from build123d import *

# Parameters (mm, degrees)
F0_W         = 185.6
F0_H         = 105.4
F1_DEPTH     = 6
F2_R         = 22.5
F3_DEPTH     = 25
F4_R         = 2
F5_T1_DEPTH  = 9
F5_S5_W      = 2
F5_S5_H      = 2
F5_T6_DEPTH  = 2
F5_S11_W     = 2
F5_S11_H     = 2
F5_T12_DEPTH = 2
F5_S17_W     = 2
F5_S17_H     = 2
F5_T18_DEPTH = 2
F5_S23_W     = 2
F5_S23_H     = 2
F5_T24_DEPTH = 2


# Not quite as in the source:
# - a fillet or chamfer that OpenCascade refuses, or shapes differently, is made with other operations: its cross-section is extruded or revolved along the edge and cut away or added


with BuildPart() as f1:
    # F0 (on Top) → F1 (new body)
    with BuildSketch(Plane.XY):
        Rectangle(F0_W, F0_H)
    extrude(amount=F1_DEPTH)

    # F2 (on face) → F3 (cut)
    with BuildSketch(Plane.XY.offset(6)):
        with Locations((50.1459216796, 0)):
            Circle(F2_R)
    extrude(amount=-F3_DEPTH, mode=Mode.SUBTRACT)

    # F4
    f4_edges = [f1.edges().sort_by_distance(p)[0] for p in [
        (0, -52.7, 6),
        (92.8, 0, 6),
        (0, 52.7, 6),
        (-92.8, 0, 6),
    ]]
    fillet(f4_edges, radius=F4_R)

    # F5: fillet of radius 2 on 4 edges, made by hand

    # F5_s2 → F5_t1 (cut)
    with BuildSketch(Plane.XY.offset(-5)):
        with BuildLine():
            ThreePointArc((92.8, -50.7), (92.2142135624, -52.1142135624), (90.8, -52.7))
            Line((90.8, -52.7), (92.8, -52.7))
            Line((92.8, -52.7), (92.8, -50.7))
        make_face()
        with BuildLine():
            ThreePointArc((92.8, 50.7), (92.2142135624, 52.1142135624), (90.8, 52.7))
            Line((90.8, 52.7), (92.8, 52.7))
            Line((92.8, 52.7), (92.8, 50.7))
        make_face()
        with BuildLine():
            ThreePointArc((-90.8, 52.7), (-92.2142135624, 52.1142135624), (-92.8, 50.7))
            Line((-92.8, 50.7), (-92.8, 52.7))
            Line((-92.8, 52.7), (-90.8, 52.7))
        make_face()
        with BuildLine():
            ThreePointArc((-90.8, -52.7), (-92.2142135624, -52.1142135624), (-92.8, -50.7))
            Line((-92.8, -50.7), (-92.8, -52.7))
            Line((-92.8, -52.7), (-90.8, -52.7))
        make_face()
    extrude(amount=F5_T1_DEPTH, mode=Mode.SUBTRACT)


with BuildPart() as f5_tool4:
    # F5_s5 → F5_t6 (new body)
    with BuildSketch(Plane.XZ.offset(50.7)):
        with Locations((-91.8, 5)):
            Rectangle(F5_S5_W, F5_S5_H)
    extrude(amount=F5_T6_DEPTH)

    # F5_s7 → F5_t8 (revolve, cut)
    with BuildSketch(Plane(origin=(-90.8, -50.7, 4), x_dir=(0.7071067812, 0, -0.7071067812), z_dir=(-0.7071067812, 0, -0.7071067812))):
        with BuildLine():
            ThreePointArc((0, -2), (2, 0), (0, 2))
            Line((0, 2), (0, -2))
        make_face()
    revolve(axis=Axis((-90.8, -50.7, 4), (0, -1, 0)), mode=Mode.SUBTRACT)


with BuildPart() as f1_1:
    add(f1.part)

    # F5_t3: cut F5_tool4
    add(f5_tool4.part, mode=Mode.SUBTRACT)


with BuildPart() as f5_tool10:
    # F5_s11 → F5_t12 (new body)
    with BuildSketch(Plane.XZ.offset(-50.7)):
        with Locations((-91.8, 5)):
            Rectangle(F5_S11_W, F5_S11_H)
    extrude(amount=-F5_T12_DEPTH)

    # F5_s13 → F5_t14 (revolve, cut)
    with BuildSketch(Plane(origin=(-90.8, 50.7, 4), x_dir=(0.7071067812, 0, -0.7071067812), z_dir=(0.7071067812, 0, 0.7071067812))):
        with BuildLine():
            ThreePointArc((0, -2), (2, 0), (0, 2))
            Line((0, 2), (0, -2))
        make_face()
    revolve(axis=Axis((-90.8, 50.7, 4), (0, 1, 0)), mode=Mode.SUBTRACT)


with BuildPart() as f1_2:
    add(f1_1.part)

    # F5_t9: cut F5_tool10
    add(f5_tool10.part, mode=Mode.SUBTRACT)


with BuildPart() as f5_tool16:
    # F5_s17 → F5_t18 (new body)
    with BuildSketch(Plane.YZ.offset(90.8)):
        with Locations((51.7, 5)):
            Rectangle(F5_S17_W, F5_S17_H)
    extrude(amount=F5_T18_DEPTH)

    # F5_s19 → F5_t20 (revolve, cut)
    with BuildSketch(Plane(origin=(90.8, 50.7, 4), x_dir=(0, -0.7071067812, -0.7071067812), z_dir=(0, -0.7071067812, 0.7071067812))):
        with BuildLine():
            ThreePointArc((0, -2), (2, 0), (0, 2))
            Line((0, 2), (0, -2))
        make_face()
    revolve(axis=Axis((90.8, 50.7, 4), (1, 0, 0)), mode=Mode.SUBTRACT)


with BuildPart() as f1_3:
    add(f1_2.part)

    # F5_t15: cut F5_tool16
    add(f5_tool16.part, mode=Mode.SUBTRACT)


with BuildPart() as f5_tool22:
    # F5_s23 → F5_t24 (new body)
    with BuildSketch(Plane.YZ.offset(90.8)):
        with Locations((-51.7, 5)):
            Rectangle(F5_S23_W, F5_S23_H)
    extrude(amount=F5_T24_DEPTH)

    # F5_s25 → F5_t26 (revolve, cut)
    with BuildSketch(Plane(origin=(90.8, -50.7, 4), x_dir=(0, 0.7071067812, -0.7071067812), z_dir=(0, -0.7071067812, -0.7071067812))):
        with BuildLine():
            ThreePointArc((0, -2), (2, 0), (0, 2))
            Line((0, 2), (0, -2))
        make_face()
    revolve(axis=Axis((90.8, -50.7, 4), (1, 0, 0)), mode=Mode.SUBTRACT)


with BuildPart() as f1_4:
    add(f1_3.part)

    # F5_t21: cut F5_tool22
    add(f5_tool22.part, mode=Mode.SUBTRACT)


solid = f1_4.part
Geometry: final body of the model. Coordinates: model frame, mm. Coordinates: 2 decimals unless noted, no trailing zeros. Order: outer loops, then holes, each group sorted by start corner. A loop starts at its lowest first (then second) coordinate and runs counter-clockwise, first axis right, second up.
(1) Draft query along Y for faces 1 (the face through (-1, 1, 0)), 2 (the face through (45.268, -21.965, 3.042)), 3 (the face through (-1, 52.7, 2)). Return one class per face: pulls with the +Y half, pulls with the -Y half, needs draft (parallel to the pull), parting line crosses it, or undercut.
(2) Material intervals for probe 1 along Y at (x, z) = (25, 4.35); probe 2 along X at (y, z) = (20, 4.2); probe 3 along X at (y, z) = (5, 2.15), sorted ascending.
(3) Section query B-B (y = 0). Return the cut outline in (x, z).
(4) Section query A-A (z = 2.3). Return the cut outline in (x, y).
(5) Section query C-C (x = 36). Return the cut outline in (y, z).
Solution:
1. face 1: needs draft
1. face 2: undercut
1. face 3: pulls with the +Y half
2. probe 1: y = -52.67 to 52.67
2. probe 2: x = -92.79 to 39.84, 60.45 to 92.79
2. probe 3: x = -92.8 to 28.21, 72.08 to 92.8
3. outline: (-92.8, 0) - (27.65, 0) - (27.65, 6) - (-90.8, 6) arc R2 ccw to (-92.8, 4) - close; (72.65, 0) - (92.8, 0) - (92.8, 4) arc R2 ccw to (90.8, 6) - (72.65, 6) - close
4. outline: (-92.8, -50.7) arc R2 ccw to (-90.8, -52.7) - (90.8, -52.7) arc R2 ccw to (92.8, -50.7) - (92.8, 50.7) arc R2 ccw to (90.8, 52.7) - (-90.8, 52.7) arc R2 ccw to (-92.8, 50.7) - close; hole circle Ø45 at (50.15, 0)
5. outline: (-52.7, 0) - (-17.5, 0) - (-17.5, 6) - (-50.7, 6) arc R2 ccw to (-52.7, 4) - close; (17.5, 0) - (52.7, 0) - (52.7, 4) arc R2 ccw to (50.7, 6) - (17.5, 6) - close
